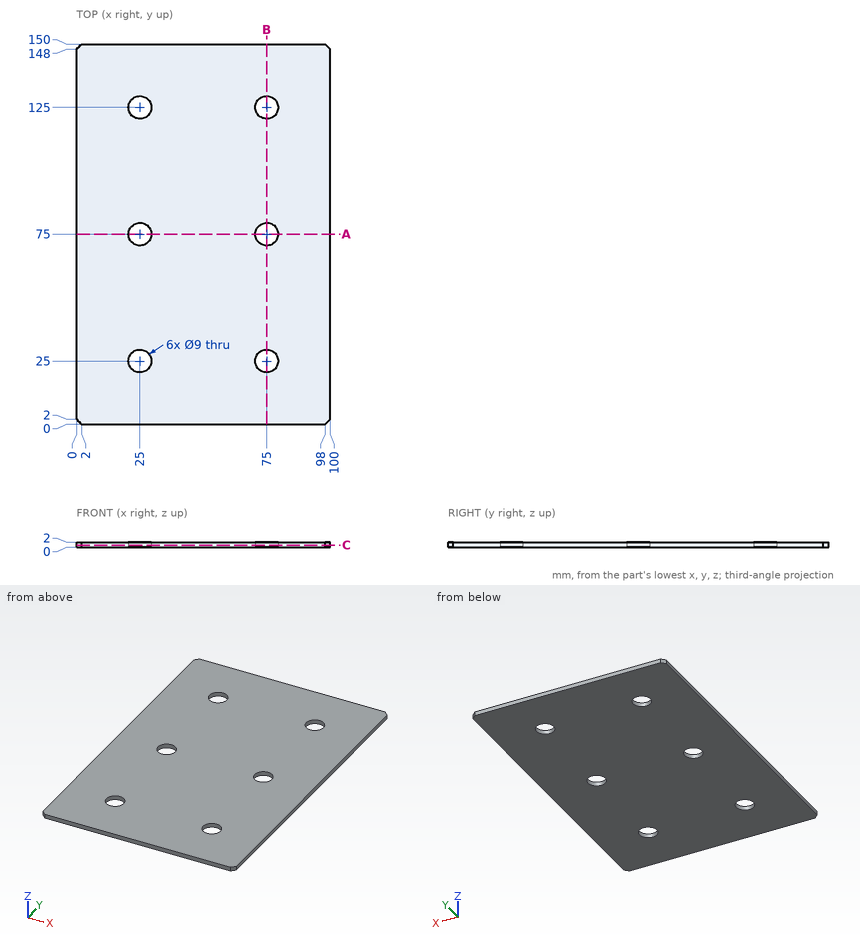
The drawing under review shows one solid part. Ordinate dimensions are in mm from its lowest x, y, z. Round coordinates to 2 decimals unless told otherwise and drop trailing zeros. Loops run counter-clockwise (first coordinate to the right, second up) from the corner with the lowest first, then second, coordinate; pieces in that order, holes last. Notation, with made-up numbers: (-19, 57) -> (4, 57) arc R29 ccw to (4, 96) -> close; hole circle Ø7 at (20, 4.5). An arc over 180 degrees is marked (long way). Answer in a Markdown table with one row per item.
1) Consider section A-A, the plane y = 75. Write out the cut boundary in (x, z).
Taken from the geometry:
| item | result |
|---|---|
| outline | (0, 0) -> (20.5, 0) -> (20.5, 2) -> (0, 2) -> close; (29.5, 0) -> (70.5, 0) -> (70.5, 2) -> (29.5, 2) -> close; (79.5, 0) -> (100, 0) -> (100, 2) -> (79.5, 2) -> close |
2) Consider section C-C, the plane z = 0.9. Write out the cut boundary in (x, y), plus the area to 3 significant figures.
Taken from the geometry:
| item | result |
|---|---|
| outline | (0, 2) -> (2, 0) -> (98, 0) -> (100, 2) -> (100, 148) -> (98, 150) -> (2, 150) -> (0, 148) -> close; hole circle Ø9 at (25, 25); hole circle Ø9 at (25, 75); hole circle Ø9 at (25, 125); hole circle Ø9 at (75, 25); hole circle Ø9 at (75, 75); hole circle Ø9 at (75, 125) |
| area | 14,600 mm² |
3) Consider section B-B, the plane x = 75. Write out the cut boundary in (y, z), plus the area to 3 significant figures.
Taken from the geometry:
| item | result |
|---|---|
| outline | (0, 0) -> (20.5, 0) -> (20.5, 2) -> (0, 2) -> close; (29.5, 0) -> (70.5, 0) -> (70.5, 2) -> (29.5, 2) -> close; (79.5, 0) -> (120.5, 0) -> (120.5, 2) -> (79.5, 2) -> close; (129.5, 0) -> (150, 0) -> (150, 2) -> (129.5, 2) -> close |
| area | 246 mm² |
4) Wall thickness on line 1 along X through (y, z) = (124.5, 0.8); line 2 along Y through (x, z) = (25, 0.6); line 3 along X through (y, z) = (23, 1.15): over which ranges is each line inside the solid? List them lowest first.
Taken from the geometry:
| item | result |
|---|---|
| line 1 | x = 0 to 20.53, 29.47 to 70.53, 79.47 to 100 |
| line 2 | y = 0 to 20.5, 29.5 to 70.5, 79.5 to 120.5, 129.5 to 150 |
| line 3 | x = 0 to 20.97, 29.03 to 70.97, 79.03 to 100 |
